Part model, mm, in its own coordinate system. Coordinates: 2 decimals unless noted, no trailing zeros. Order: outer loops, then holes, each group sorted by start corner. A loop starts at its lowest first (then second) coordinate and runs counter-clockwise, first axis right, second up.
from build123d import *

# Parameters (mm, degrees)
BOSS_EXTRUDE1_DEPTH = 20
FILLET2_R           = 12


with BuildPart() as part:
    # Sketch1 → Boss-Extrude1 (new body)
    with BuildSketch(Plane(origin=(0, 0, 0), x_dir=(1, 0, 0), z_dir=(0, 1, 0))):
        with BuildLine():
            Line((-24.659328932, -13.476609998), (-24.659328932, 13.476609998))
            Line((-24.659328932, 13.476609998), (-49.318657865, 13.476609998))
            Line((-49.318657865, 13.476609998), (-43.570374654, 7.193602767))
            ThreePointArc((-43.570374654, 7.193602767), (-33.058724148, 8.9227509), (-27.238993399, 0))
            ThreePointArc((-27.238993399, 0), (-28.066242499, -3.93026925), (-30.407612143, -7.193602767))
            Line((-30.407612143, -7.193602767), (-24.659328932, -13.476609998))
        make_face()
        with BuildLine():
            Line((-49.318657865, -13.476609998), (-24.659328932, -13.476609998))
            Line((-24.659328932, -13.476609998), (-30.407612143, -7.193602767))
            ThreePointArc((-30.407612143, -7.193602767), (-44.182596166, -6.581381255), (-43.570374654, 7.193602767))
            Line((-43.570374654, 7.193602767), (-49.318657865, 13.476609998))
            Line((-49.318657865, 13.476609998), (-49.318657865, -13.476609998))
        make_face()
        with BuildLine():
            Line((0, -13.476609998), (0, 13.476609998))
            Line((0, 13.476609998), (-24.659328932, 13.476609998))
            Line((-24.659328932, 13.476609998), (-18.911045721, 7.193602767))
            ThreePointArc((-18.911045721, 7.193602767), (-8.399395216, 8.9227509), (-2.579664466, 0))
            ThreePointArc((-2.579664466, 0), (-3.406913566, -3.93026925), (-5.748283211, -7.193602767))
            Line((-5.748283211, -7.193602767), (0, -13.476609998))
        make_face()
        with BuildLine():
            Line((-24.659328932, -13.476609998), (0, -13.476609998))
            Line((0, -13.476609998), (-5.748283211, -7.193602767))
            ThreePointArc((-5.748283211, -7.193602767), (-19.523267233, -6.581381255), (-18.911045721, 7.193602767))
            Line((-18.911045721, 7.193602767), (-24.659328932, 13.476609998))
            Line((-24.659328932, 13.476609998), (-24.659328932, -13.476609998))
        make_face()
        with BuildLine():
            Line((24.659328932, 13.476609998), (0, 13.476609998))
            Line((0, 13.476609998), (5.748283211, 7.193602767))
            ThreePointArc((5.748283211, 7.193602767), (16.259933717, 8.9227509), (22.079664466, 0))
            ThreePointArc((22.079664466, 0), (21.252415366, -3.93026925), (18.911045721, -7.193602767))
            Line((18.911045721, -7.193602767), (24.659328932, -13.476609998))
            Line((24.659328932, -13.476609998), (24.659328932, 13.476609998))
        make_face()
        with BuildLine():
            Line((5.748283211, 7.193602767), (0, 13.476609998))
            Line((0, 13.476609998), (0, -13.476609998))
            Line((0, -13.476609998), (24.659328932, -13.476609998))
            Line((24.659328932, -13.476609998), (18.911045721, -7.193602767))
            ThreePointArc((18.911045721, -7.193602767), (5.136061699, -6.581381255), (5.748283211, 7.193602767))
        make_face()
        with BuildLine():
            Line((49.318657865, 13.476609998), (24.659328932, 13.476609998))
            Line((24.659328932, 13.476609998), (30.407612143, 7.193602767))
            ThreePointArc((30.407612143, 7.193602767), (40.919262649, 8.9227509), (46.738993399, 0))
            ThreePointArc((46.738993399, 0), (45.911744298, -3.93026925), (43.570374654, -7.193602767))
            Line((43.570374654, -7.193602767), (49.318657865, -13.476609998))
            Line((49.318657865, -13.476609998), (49.318657865, 13.476609998))
        make_face()
        with BuildLine():
            Line((30.407612143, 7.193602767), (24.659328932, 13.476609998))
            Line((24.659328932, 13.476609998), (24.659328932, -13.476609998))
            Line((24.659328932, -13.476609998), (49.318657865, -13.476609998))
            Line((49.318657865, -13.476609998), (43.570374654, -7.193602767))
            ThreePointArc((43.570374654, -7.193602767), (29.795390631, -6.581381255), (30.407612143, 7.193602767))
        make_face()
    extrude(amount=BOSS_EXTRUDE1_DEPTH)

    # Fillet2
    fillet2_edges = [part.edges().sort_by_distance(p)[0] for p in [
        (-49.318657865, 10, 13.476609998),
        (-49.318657865, 10, -13.476609998),
        (49.318657865, 10, -13.476609998),
        (49.318657865, 10, 13.476609998),
    ]]
    fillet(fillet2_edges, radius=FILLET2_R)


solid = part.part
Q1. Pin check, flat tips, straight feed: pin 1 Ø1.5 at (y, z) = (3, -7) entering from -X; pin 2 Ø1 at (y, z) = (15.5, 3) entering from -X. Stop position of each tip, or through.
Results list:
pin 1: stops at x = -48.33
pin 2: stops at x = -49.27
Q2. Cut at A-A on y = 15.75. Write the cut outline in (x, z).
Results list:
outline: (-49.32, -1.48) arc R12 ccw to (-37.32, -13.48) - (37.32, -13.48) arc R12 ccw to (49.32, -1.48) - (49.32, 1.48) arc R12 ccw to (37.32, 13.48) - (-37.32, 13.48) arc R12 ccw to (-49.32, 1.48) - close; hole circle Ø19.5 at (-36.99, 0); hole circle Ø19.5 at (-12.33, 0); hole circle Ø19.5 at (12.33, 0); hole circle Ø19.5 at (36.99, 0)
Q3. Cut at B-B on z = -3. Write the cut outline in (x, y).
Results list:
outline: (-49.22, 0) - (-46.27, 0) - (-46.27, 20) - (-49.22, 20) - close; (-27.71, 0) - (-21.61, 0) - (-21.61, 20) - (-27.71, 20) - close; (-3.05, 0) - (3.05, 0) - (3.05, 20) - (-3.05, 20) - close; (21.61, 0) - (27.71, 0) - (27.71, 20) - (21.61, 20) - close; (46.27, 0) - (49.22, 0) - (49.22, 20) - (46.27, 20) - close
Q4. Wall check: line 1 along X through (y, z) = (14.5, 6); line 2 along X through (y, z) = (9, 8.75); line 3 along Z through (x, y) = (37, 17.25). Give the ranges that are in metal, low to high.
Results list:
line 1: x = -48.43 to -44.67, -29.3 to -20.01, -4.64 to 4.64, 20.01 to 29.3, 44.67 to 48.43
line 2: x = -46.86 to -41.29, -32.69 to -16.63, -8.03 to 8.03, 16.63 to 32.69, 41.29 to 46.86
line 3: z = -13.48 to -9.75, 9.75 to 13.48
